Design review of the part built by this model. Coordinates are the model's own, in mm. Face numbers are marked on the shaded views. A direction names the side the tool comes from. Coordinates: 2 decimals unless noted, no trailing zeros. Order: outer loops, then holes, each group sorted by start corner. A loop starts at its lowest first (then second) coordinate and runs counter-clockwise, first axis right, second up. Notation, with made-up numbers: M -14.5,0 L 10.5,0 A4 ccw 10.5,4 Z; hole C 10.5,25 d3. An arc over 180 degrees is marked long. Answer as a JSON object with one key per item and string values.
from build123d import *

# Parameters (mm, degrees)
BOSS_EXTRUDE4_DEPTH = 3
SKETCH5_R           = 1.4
BOSS_EXTRUDE5_DEPTH = 4.6
SKETCH6_R           = 2.25
BOSS_EXTRUDE6_DEPTH = 0.4


with BuildPart() as part:
    # Sketch4 → Boss-Extrude4 (new body, symmetric)
    with BuildSketch(Plane(origin=(0, 0, 0), x_dir=(0, 0, -1), z_dir=(1, 0, 0))):
        Polygon((-5, -1), (-5, 0.8), (-2.6, 0.8), (-2.6, 0), (2.6, 0), (2.6, 0.8), (5, 0.8), (5, -1), (9.5, -1), (9.5, -2.2), (4.2, -2.2), (4.2, 0), (3.4, 0), (3.4, -0.8), (-3.4, -0.8), (-3.4, 0), (-4.2, 0), (-4.2, -2.2), (-9.5, -2.2), (-9.5, -1), align=None)
    extrude(amount=BOSS_EXTRUDE4_DEPTH, both=True)

    # Sketch5 → Boss-Extrude5 (add)
    with BuildSketch(Plane(origin=(0, -1, 0), x_dir=(1, 0, 0), z_dir=(0, 1, 0))):
        with Locations((0, -7)):
            Circle(SKETCH5_R)
        with Locations((0, 7)):
            Circle(SKETCH5_R)
    extrude(amount=-BOSS_EXTRUDE5_DEPTH)

    # Sketch6 → Boss-Extrude6 (add)
    with BuildSketch(Plane.XZ.offset(5.6)):
        with Locations((0, -7)):
            Circle(SKETCH6_R)
        with Locations((0, 7)):
            Circle(SKETCH6_R)
    extrude(amount=BOSS_EXTRUDE6_DEPTH)


solid = part.part
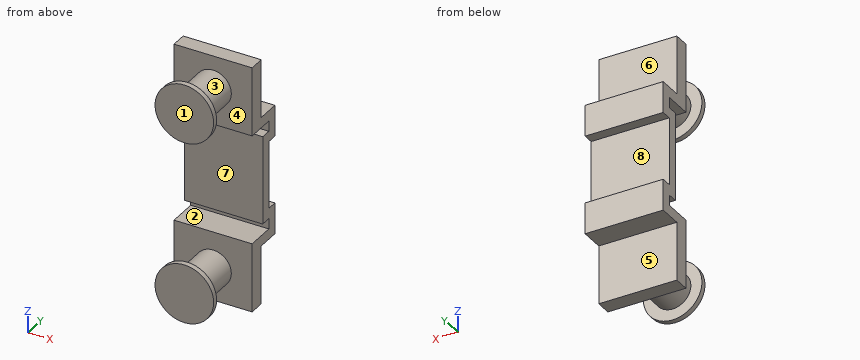
1) Add section C-C (x = -1.9). State the section outline as (y, z) points.
Taken from the geometry:
{"outline": "M -6,-8.21 L -5.6,-8.21 L -5.6,-5.79 L -6,-5.79 Z; M -6,5.79 L -5.6,5.79 L -5.6,8.21 L -6,8.21 Z; M -2.2,-9.5 L -1,-9.5 L -1,-5 L 0.8,-5 L 0.8,-2.6 L 0,-2.6 L 0,2.6 L 0.8,2.6 L 0.8,5 L -1,5 L -1,9.5 L -2.2,9.5 L -2.2,4.2 L 0,4.2 L 0,3.4 L -0.8,3.4 L -0.8,-3.4 L 0,-3.4 L 0,-4.2 L -2.2,-4.2 Z"}
2) Add section B-B (z = -7). State the section outline as (x, y) points, and give its area (3 significant figures).
Taken from the geometry:
{"outline": "M -3,-2.2 L -1.4,-2.2 L -1.4,-5.6 L -2.25,-5.6 L -2.25,-6 L 2.25,-6 L 2.25,-5.6 L 1.4,-5.6 L 1.4,-2.2 L 3,-2.2 L 3,-1 L -3,-1 Z", "area": "18.5 mm2"}
3) Add section D-D (y = -4.25). State the section outline as (x, z) points, and give its area (3 significant figures).
Taken from the geometry:
{"outline": "C 0,-7 d2.8; C 0,7 d2.8", "area": "12.3 mm2"}
4) Tool access review of the marked faces 4, 5, 6, 7 and 8: name each direction out of +Z, -Z, +X, -X, +Y, -Y from which nothing blocks a thin tool from reaching the whole face with its end or side.
Taken from the geometry:
{"face 4": "none", "face 5": "-Z, +X, -X, +Y", "face 6": "+Z, +X, -X, +Y", "face 7": "+X, -X, -Y", "face 8": "+X, -X, +Y"}
5) To check wall thickness, follow L1, parallel to Z at x = -0.25, y = 0.5; L2, parallel to Y at x = 1.55, z = -8.25; L3, parallel to Y at x = 1.25, z = -1.75. State the ranges of each line that lie inside material, in increasing order.
Taken from the geometry:
{"L1": "z = -5 to -2.6, 2.6 to 5", "L2": "y = -6 to -5.6, -2.2 to -1", "L3": "y = -0.8 to 0"}
6) Add section A-A (y = -1.5). State the section outline as (x, z) points.
Taken from the geometry:
{"outline": "M -3,-9.5 L 3,-9.5 L 3,-4.2 L -3,-4.2 Z; M -3,4.2 L 3,4.2 L 3,9.5 L -3,9.5 Z"}
7) Insertion check: pin 1 Ø1.6 at (x, z) = (1.5, -1) entering from +Y; pin 2 Ø0.5 at (x, y) = (0, 0.5) entering from -Z; pin 3 Ø2 at (x, z) = (1.5, -7.5) entering from +Y. Each pin has a flat end and moves straight along its axis. Give the tip position at first contact, or say it passes through.
Taken from the geometry:
{"pin 1": "stops at y = 0", "pin 2": "stops at z = -5", "pin 3": "stops at y = -1"}
8) Mouldability with a two-part tool opening along Z and no side actions: class the marked faces 1, 2 and 3 as released by +Z, released by -Z, zero draft, split by the parting line, or undercut.
Taken from the geometry:
{"face 1": "zero draft", "face 2": "undercut", "face 3": "undercut"}
